Geometry: final body of the model. Coordinates: model frame, mm. Round coordinates to 2 decimals unless told otherwise and drop trailing zeros. Write each loop counter-clockwise with the first axis right and the second up, starting at its lowest first coordinate (ties: lowest second). Pieces come first, ordered by that corner, then holes. Notation, with made-up numbers: (-18, 40.5) - (29, 40.5) arc R21 ccw to (29, 75.5) - close; hole circle Ø1 at (-38.75, 74). An arc over 180 degrees is marked (long way). Write each question's results on one line, items separated by ' | '.
from build123d import *

# Parameters (mm, degrees)
F0_R     = 11.2
F1_DEPTH = 7


with BuildPart() as f1:
    # F0 (on Top) → F1 (new body)
    with BuildSketch(Plane.XY):
        with BuildLine():
            ThreePointArc((23.30928, -0.214358), (12.611296, 7.857897), (11.960537, 21.243885))
            ThreePointArc((11.960537, 21.243885), (12.093594, 21.558476), (12.23342, 21.870118))
            ThreePointArc((12.23342, 21.870118), (-0.876031, 39.999186), (-11.469, 20.293608))
            ThreePointArc((-11.469, 20.293608), (-13.110787, 6.992755), (-24.378013, -0.263813))
            ThreePointArc((-24.378013, -0.263813), (-24.716985, -0.305878), (-25.056787, -0.340607))
            ThreePointArc((-25.056787, -0.340607), (-34.202296, -20.758258), (-11.84028, -20.079249))
            ThreePointArc((-11.84028, -20.079249), (0.49949, -14.850652), (12.417475, -20.980072))
            ThreePointArc((12.417475, -20.980072), (12.623391, -21.252598), (12.823368, -21.529511))
            ThreePointArc((12.823368, -21.529511), (35.078326, -19.240928), (23.30928, -0.214358))
        make_face()
        with Locations((-23.233978, -13.414144)):
            Circle(F0_R, mode=Mode.SUBTRACT)
        with Locations((23.233978, -13.414144)):
            Circle(F0_R, mode=Mode.SUBTRACT)
        Circle(F0_R, mode=Mode.SUBTRACT)
        with Locations((0, 26.828287)):
            Circle(F0_R, mode=Mode.SUBTRACT)
    extrude(amount=F1_DEPTH)


solid = f1.part
Q1. Mould query, pull axis Y, two halves, no side actions, for faces 1 (the cylindrical face through (-2.428, 15.895, 3.451)), 2 (the cylindrical face through (-0.5, 40.02, 3.45)), 3 (the cylindrical face through (0.306, -14.845, 3.451)), 4 (the flat face through (5.2, -10.4, 0)). Classes: pulls with the +Y half, pulls with the -Y half, needs draft (parallel to the pull), parting line crosses it, or undercut.
Answer block:
face 1: undercut | face 2: undercut | face 3: pulls with the -Y half | face 4: needs draft
Q2. Section query D-D, the plane y = 12. Return loops of the section in (x, z).
Answer block:
outline: (-11.06, 0) - (11.11, 0) - (11.11, 7) - (-11.06, 7) - close
Q3. Section query B-B, the plane z = 1.75. Return loops of the section in (x, y).
Answer block:
outline: (-25.06, -0.34) arc R13.2 ccw (long way) to (-11.84, -20.08) arc R15.8 cw to (12.42, -20.98) arc R15.8 cw to (12.82, -21.53) arc R13.2 ccw (long way) to (23.31, -0.21) arc R15.8 cw to (11.96, 21.24) arc R15.8 cw to (12.23, 21.87) arc R13.2 ccw (long way) to (-11.47, 20.29) arc R15.8 cw to (-24.38, -0.26) arc R15.8 cw to start; hole circle Ø22.4 at (-23.23, -13.41); hole circle Ø22.4 at (0, 0); hole circle Ø22.4 at (0, 26.83); hole circle Ø22.4 at (23.23, -13.41)
Q4. Ray query, line 1 along Y through (x, z) = (0, 2); line 2 along X through (y, z) = (-7.5, 3.75); line 3 along Y through (x, z) = (7.5, 6). Return the intervals inside material, ascending.
Answer block:
line 1: -14.84 to -11.2, 11.2 to 15.63, 38.03 to 40.03 | line 2: -35.03 to -32.75, -13.72 to -8.32, 8.32 to 13.72, 32.75 to 35.03 | line 3: -16.78 to -8.32, 8.32 to 18.51, 35.15 to 37.69
Q5. Pin query (flat end, axial travel): pin 1 (2 mm diameter, centred on x = 4.5, z = 5, fed in from +Y); pin 2 (2 mm diameter, centred on y = 26.5, z = 3, fed in from +X); pin 3 (1.5 mm diameter, centred on y = 5, z = 1.5, fed in from +X). Return the tip coordinate at first contact, or that it passes through.
Answer block:
pin 1: y = 39.56 | pin 2: x = 13.2 | pin 3: x = 15.23
Q6. Section query C-C, the plane x = -18. Return loops of the section in (y, z), plus the area to 3 significant figures.
Answer block:
outline: (-25.53, 0) - (-23.32, 0) - (-23.32, 7) - (-25.53, 7) - close; (-3.51, 0) - (2.07, 0) - (2.07, 7) - (-3.51, 7) - close | area: 54.6 mm2
Q7. Section query A-A, the plane x = 0. Return loops of the section in (y, z).
Answer block:
outline: (-14.84, 0) - (-11.2, 0) - (-11.2, 7) - (-14.84, 7) - close; (11.2, 0) - (15.63, 0) - (15.63, 7) - (11.2, 7) - close; (38.03, 0) - (40.03, 0) - (40.03, 7) - (38.03, 7) - close
